```python
from build123d import *

# Parameters (mm, degrees)
F1_DEPTH  = 50
F2_R      = 2.5
F3_R      = 9
F4_DEPTH  = 100
F6_START  = -33
F5_R      = 12
F6_DEPTH  = 34
F7_R      = 5
F9_DEPTH  = 3
F8_R      = 3
F10_DEPTH = 2.5


with BuildPart() as f1:
    # F0 (on Front) → F1 (new body, symmetric)
    with BuildSketch(Plane.XZ):
        with BuildLine():
            Line((27.5, 5.5), (0, 5.5))
            Line((0, 5.5), (0, 0))
            Line((0, 0), (37.3689500386, 0))
            Line((37.3689500386, 0), (38.25, 0.8810499614))
            ThreePointArc((38.25, 0.8810499614), (33.172918626, 3.6252742871), (29.9640842591, 8.4222425415))
            ThreePointArc((29.9640842591, 8.4222425415), (29.4112308016, 6.388417913), (27.5, 5.5))
        make_face()
        with BuildLine():
            ThreePointArc((53.25, 12.5), (39.1800952788, 24.320130898), (29.9640842591, 8.4222425415))
            ThreePointArc((29.9640842591, 8.4222425415), (33.172918626, 3.6252742871), (38.25, 0.8810499614))
            ThreePointArc((38.25, 0.8810499614), (48.5984692283, 3.0131670195), (53.25, 12.5))
        make_face()
    extrude(amount=F1_DEPTH, both=True)

    # F2
    f2_edges = [f1.edges().sort_by_distance(p)[0] for p in [
        (0, 0, 5.5),
    ]]
    fillet(f2_edges, radius=F2_R)

    # F3 (on face) → F4 (cut, through all)
    with BuildSketch(Plane.XZ.offset(50)):
        with Locations((41.25, 12.5)):
            Circle(F3_R)
    extrude(amount=-F4_DEPTH, mode=Mode.SUBTRACT)

    # F5 (on face) → F6 (cut)
    with BuildSketch(Plane.XZ.offset(50).offset(F6_START)):
        with Locations((41.25, 12.5)):
            Circle(F5_R)
    extrude(amount=-F6_DEPTH, mode=Mode.SUBTRACT)

    # F7 (on face) → F9 (cut)
    with BuildSketch(Plane.XY.offset(5.5)):
        with Locations((15, 0)):
            Circle(F7_R)
        with Locations((15, 37)):
            Circle(F7_R)
        with Locations((15, -37)):
            Circle(F7_R)
    extrude(amount=-F9_DEPTH, mode=Mode.SUBTRACT)

    # F8 (on face) → F10 (cut, through all)
    with BuildSketch(Plane(origin=(0, 0, 0), x_dir=(1, 0, 0), z_dir=(0, 0, -1))):
        with Locations((15, -37)):
            Circle(F8_R)
        with Locations((15, 0)):
            Circle(F8_R)
        with Locations((15, 37)):
            Circle(F8_R)
    extrude(amount=-F10_DEPTH, mode=Mode.SUBTRACT)


solid = f1.part
```
Here's how the part is built. I have some questions about the finished solid (model axes, mm). A direction names the side the tool comes from. Coordinates: 2 decimals unless noted, no trailing zeros. Loops run counter-clockwise (first coordinate to the right, second up) from the corner with the lowest first, then second, coordinate; pieces in that order, holes last. Notation, with made-up numbers: (56, -20.5) - (115, -20.5) arc R29 cw to (115, 15.5) - close; hole circle Ø11 at (32.25, -2). An arc over 180 degrees is marked (long way). Answer as CSV lines item,"result".
Q1. If we section it at D-D, the plane z = 4.5: Write out the boundary of the cut face in (x, y), and give its area (3 significant figures).
Response:
outline,"(0.5, -50) - (37.13, -50) - (37.13, -17) - (32.31, -17) - (32.31, 17) - (37.13, 17) - (37.13, 50) - (0.5, 50) - close; (45.37, -50) - (50.19, -50) - (50.19, -17) - (45.37, -17) - close; (45.37, 17) - (50.19, 17) - (50.19, 50) - (45.37, 50) - close; hole circle Ø10 at (15, -37); hole circle Ø10 at (15, 0); hole circle Ø10 at (15, 37)"
area,"3,580 mm2"
Q2. For pin 1 (9.5 mm diameter, centred on x = 15, y = 37, fed in from +Z); pin 2 (3 mm diameter, centred on x = 33.5, y = 32, fed in from +Z); pin 3 (6 mm diameter, centred on x = 11, y = -39.5, fed in from +Z), each with a flat end and sliding along its axis, tell me the tip position at first contact or that it passes through.
Response:
pin 1,"z = 2.5"
pin 2,"z = 22.74"
pin 3,"z = 5.5"
Q3. If I drill on L1, parallel to Y at x = 15, z = 1.4; L2, parallel to Y at x = 15, z = 3.7; L3, parallel to X at y = -29, z = 13, over which ranges is the centre line in solid material (lowest first)? Write a range as [from, to].
Response:
L1,"[-50, -40], [-34, -3], [3, 34], [40, 50]"
L2,"[-50, -42], [-32, -5], [5, 32], [42, 50]"
L3,"[29.26, 32.26], [50.24, 53.24]"
Q4. If we section it at C-C, the plane y = 0: Write out the boundary of the cut face in (x, z), and give its area (3 significant figures).
Response:
outline,"(0, 0) - (12, 0) - (12, 2.5) - (10, 2.5) - (10, 5.5) - (2.5, 5.5) arc R2.5 ccw to (0, 3) - close; (18, 0) - (37.37, 0) - (38.25, 0.88) arc R12 cw to (29.96, 8.42) arc R2.5 cw to (27.5, 5.5) - (20, 5.5) - (20, 2.5) - (18, 2.5) - close"
area,"147 mm2"
Q5. For faces 5 (the face through (12, 0, 1)), 6 (the face through (19.77, -35.5, 4.02)), 7 (the face through (33.113, -0.238, 3.68)), which set-ups out of +Z, -Z, +X, -X, +Y, -Y let a thin tool reach every point of the face, with its end or its side?
Response:
face 5,"+Z, -Z"
face 6,"+Z"
face 7,"+Z, +X"
Q6. We'd pull the mould along X, two halves only. Please class faces 1 (the face through (9.6, -0.7, 5.5)), 2 (the face through (14.9, -3.3, 2.5)), 3 (the face through (0, -1, 2)), 4 (the face through (12.79, 34.97, 1.23)): pulls with the +X half, pulls with the -X half, needs draft (parallel to the pull), parting line crosses it, or undercut.
Response:
face 1,"needs draft"
face 2,"undercut"
face 3,"pulls with the -X half"
face 4,"undercut"
Q7. If we section it at A-A, the plane y = -37: Write out the boundary of the cut face in (x, z), and give its area (3 significant figures).
Response:
outline,"(0, 0) - (12, 0) - (12, 2.5) - (10, 2.5) - (10, 5.5) - (2.5, 5.5) arc R2.5 ccw to (0, 3) - close; (18, 0) - (37.37, 0) - (38.25, 0.88) arc R12 ccw (long way) to (29.96, 8.42) arc R2.5 cw to (27.5, 5.5) - (20, 5.5) - (20, 2.5) - (18, 2.5) - close; hole circle Ø18 at (41.25, 12.5)"
area,"345 mm2"
Q8. If we section it at B-B, the plane x = 41.25: Write out the boundary of the cut face in (y, z).
Response:
outline,"(-50, 0.5) - (-17, 0.5) - (-17, 3.5) - (-50, 3.5) - close; (-50, 21.5) - (-17, 21.5) - (-17, 24.5) - (-50, 24.5) - close; (17, 0.5) - (50, 0.5) - (50, 3.5) - (17, 3.5) - close; (17, 21.5) - (50, 21.5) - (50, 24.5) - (17, 24.5) - close"
